Design review of the part built by this model. Coordinates are the model's own, in mm. Face numbers are marked on the shaded views. A direction names the side the tool comes from. Coordinates: 2 decimals unless noted, no trailing zeros. Loops run counter-clockwise (first coordinate to the right, second up) from the corner with the lowest first, then second, coordinate; pieces in that order, holes last. Notation, with made-up numbers: (-37.5, 10.25) -> (-28.5, 10.25) arc R10 cw to (-28.5, 24.25) -> close; hole circle Ø7 at (-7.75, 7). An arc over 180 degrees is marked (long way). One line per item, written item: value. Start each with the question number.
1. Add section B-B on z = 0.75. Write out the cut boundary in (x, y).
2. Draft analysis for pull direction Z (two halves, no side actions). For the marked faces 4, 5 and 6, state which applies: pulls with the +Z half, pulls with the -Z half, needs draft (parallel to the pull), parting line crosses it, or undercut.
3. Insertion check: pin 1 (1 mm diameter, centred on y = -4.5, z = 0, fed in from -X); pin 2 (3 mm diameter, centred on y = -11, z = 0, fed in from +X); pin 3 (4 mm diameter, centred on x = 4.5, z = 1, fed in from -Y); pin 4 (2 mm diameter, centred on x = -2.5, z = -0.5, fed in from -Y). Each pin has a flat end and moves straight along its axis. Give the tip position at first contact, or say it passes through.
4. Add section A-A on x = 0. Write out the cut boundary in (y, z).
5. For probe 1 along X at (y, z) = (-0.95, 0); probe 2 along Y at (x, z) = (5, -1.25), list the stretches that pass through material, from the lowest coordinate up.
6. Machinability: for the marked faces 1, 2 and 3, which of the approach directions +Z, -Z, +X, -X, +Y, -Y give a long, thin tool a straight path to every point of the face, cutting with its end or side? Answer none if there is none.
7. Add section C-C on x = -4.5. Write out the cut boundary in (y, z).
```python
from build123d import *

# Parameters (mm, degrees)
PAD_DEPTH         = 3.9
PAD001_DEPTH      = 7.8
SKETCH002_R       = 1.75
POCKET_DEPTH      = 4.001
POCKET_DEPTH_BACK = 12.001
POCKET001_DEPTH   = 4
SKETCH004_R       = 3
POCKET002_DEPTH   = 6
SKETCH005_W       = 1.2
SKETCH005_H       = 5
POCKET003_DEPTH   = 16.001
SKETCH006_W       = 2
SKETCH006_H       = 5
POCKET004_DEPTH   = 17.401
FILLET_R          = 3.7
FILLET001_R       = 1.19


with BuildPart() as part:
    # Sketch → Pad (new body, symmetric)
    with BuildSketch(Plane.XY):
        with BuildLine():
            Line((-3.9, 0), (3.9, 0))
            Line((3.9, 0), (3.9, 0.8))
            Line((3.9, 0.8), (5.35, 0.8))
            ThreePointArc((5.35, 0.8), (0, 4), (-5.35, 0.8))
            Line((-5.35, 0.8), (-3.9, 0.8))
            Line((-3.9, 0.8), (-3.9, 0))
        make_face()
    extrude(amount=PAD_DEPTH, both=True)

    # Sketch001 (on Face7 of Pad) → Pad001 (join)
    with BuildSketch(Plane(origin=(0, 0, -3.9), x_dir=(1, 0, 0), z_dir=(0, 0, -1))):
        with BuildLine():
            Line((-8.7, 12), (-8.7, 8))
            Line((-8.7, 8), (-3.9, 3.5))
            Line((-3.9, 3.5), (-3.9, 0))
            Line((-3.9, 0), (3.9, 0))
            Line((3.9, 3.5), (3.9, 0))
            Line((8.7, 8), (3.9, 3.5))
            Line((8.7, 8), (8.7, 12))
            Line((8.7, 12), (5.5, 12))
            ThreePointArc((-5.5, 12), (0, 6.5), (5.5, 12))
            Line((-5.5, 12), (-8.7, 12))
        make_face()
    extrude(amount=-PAD001_DEPTH)

    # Sketch002 → Pocket (cut, two sides)
    with BuildSketch(Plane.XZ) as pocket_sk:
        Circle(SKETCH002_R)
    extrude(amount=-POCKET_DEPTH, mode=Mode.SUBTRACT)
    extrude(pocket_sk.sketch, amount=POCKET_DEPTH_BACK, mode=Mode.SUBTRACT)

    # Sketch003 (on DatumPlane) → Pocket001 (cut)
    with BuildSketch(Plane.XZ.offset(-4)):
        Polygon((-1.6, -2.771281), (1.6, -2.771281), (3.2, 0), (1.6, 2.771281), (-1.6, 2.771281), (-3.2, 0), align=None)
    extrude(amount=POCKET001_DEPTH, mode=Mode.SUBTRACT)

    # Sketch004 (on DatumPlane) → Pocket002 (cut)
    with BuildSketch(Plane.XZ.offset(3)):
        Circle(SKETCH004_R)
    extrude(amount=POCKET002_DEPTH, mode=Mode.SUBTRACT)

    # Sketch005 (on Face22 of Pocket002) → Pocket003 (cut, through all)
    with BuildSketch(Plane.XZ.offset(12)):
        with Locations((-8.1, 0)):
            Rectangle(SKETCH005_W, SKETCH005_H)
        with Locations((8.1, 0)):
            Rectangle(SKETCH005_W, SKETCH005_H)
    extrude(amount=-POCKET003_DEPTH, mode=Mode.SUBTRACT)

    # Sketch006 (on Face23 of Pocket003) → Pocket004 (cut, through all)
    with BuildSketch(Plane.YZ.offset(8.7)):
        with Locations((-7, 0)):
            Rectangle(SKETCH006_W, SKETCH006_H)
    extrude(amount=-POCKET004_DEPTH, mode=Mode.SUBTRACT)

    # Fillet
    fillet_edges = [part.edges().sort_by_distance(p)[0] for p in [
        (-3.9, -1.75, 3.9),
        (-3.9, -1.75, -3.9),
        (3.9, -1.75, 3.9),
        (3.9, -1.75, -3.9),
    ]]
    fillet(fillet_edges, radius=FILLET_R)

    # Fillet001
    fillet001_edges = [part.edges().sort_by_distance(p)[0] for p in [
        (7.5, -10, 2.5),
        (7.5, -10, -2.5),
        (-7.5, -10, 2.5),
        (-7.5, -10, -2.5),
    ]]
    fillet(fillet001_edges, radius=FILLET001_R)


solid = part.part
```
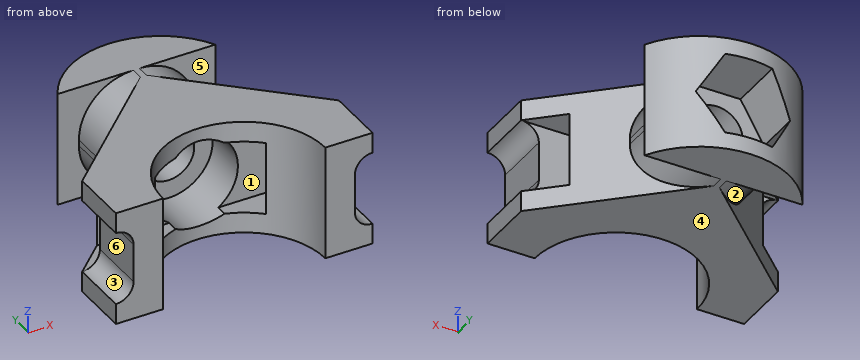
Worked answers:
1. outline: (-7.5, -12) -> (-5.5, -12) arc R5.5 cw to (-3.77, -8) -> (-7.5, -8) -> close; (-6.57, -6) -> (-2.9, -6) -> (-2.9, -3) -> (-1.58, -3) -> (-1.58, 0) -> (-2.77, 0) -> (-2.77, 3.33) arc R6.07 ccw to (-5.35, 0.8) -> (-3.86, 0.8) -> (-3.86, -3.46) -> close; (1.58, -3) -> (2.9, -3) -> (2.9, -6) -> (6.57, -6) -> (3.86, -3.46) -> (3.86, 0.8) -> (5.35, 0.8) arc R6.07 ccw to (2.77, 3.33) -> (2.77, 0) -> (1.58, 0) -> close; (3.77, -8) arc R5.5 cw to (5.5, -12) -> (7.5, -12) -> (7.5, -8) -> close
2. face 4: pulls with the -Z half
2. face 5: needs draft
2. face 6: undercut
3. pin 1: stops at x = -5.5
3. pin 2: stops at x = 7.52
3. pin 3: stops at y = -12
3. pin 4: stops at y = -6
4. outline: (-6.5, -3.9) -> (4, -3.9) -> (4, -2.77) -> (0, -2.77) -> (0, -1.75) -> (-3, -1.75) -> (-3, -3) -> (-6.5, -3) -> close; (-6.5, 3) -> (-3, 3) -> (-3, 1.75) -> (0, 1.75) -> (0, 2.77) -> (4, 2.77) -> (4, 3.9) -> (-6.5, 3.9) -> close
5. probe 1: x = -3.9 to -1.75, 1.75 to 3.9
5. probe 2: y = -9.71 to -8, -6 to -4.53, 0.8 to 1.37
6. face 1: +X, -X
6. face 2: -Z, -X
6. face 3: -X, +Y, -Y
7. outline: (-8.84, -3.9) -> (-4.06, -3.9) -> (-4.06, 3.9) -> (-8.84, 3.9) -> close; (0.8, -3.9) -> (2, -3.9) -> (2, 3.9) -> (0.8, 3.9) -> close; hole (-8, -2.5) -> (-6, -2.5) -> (-6, 2.5) -> (-8, 2.5) -> close
